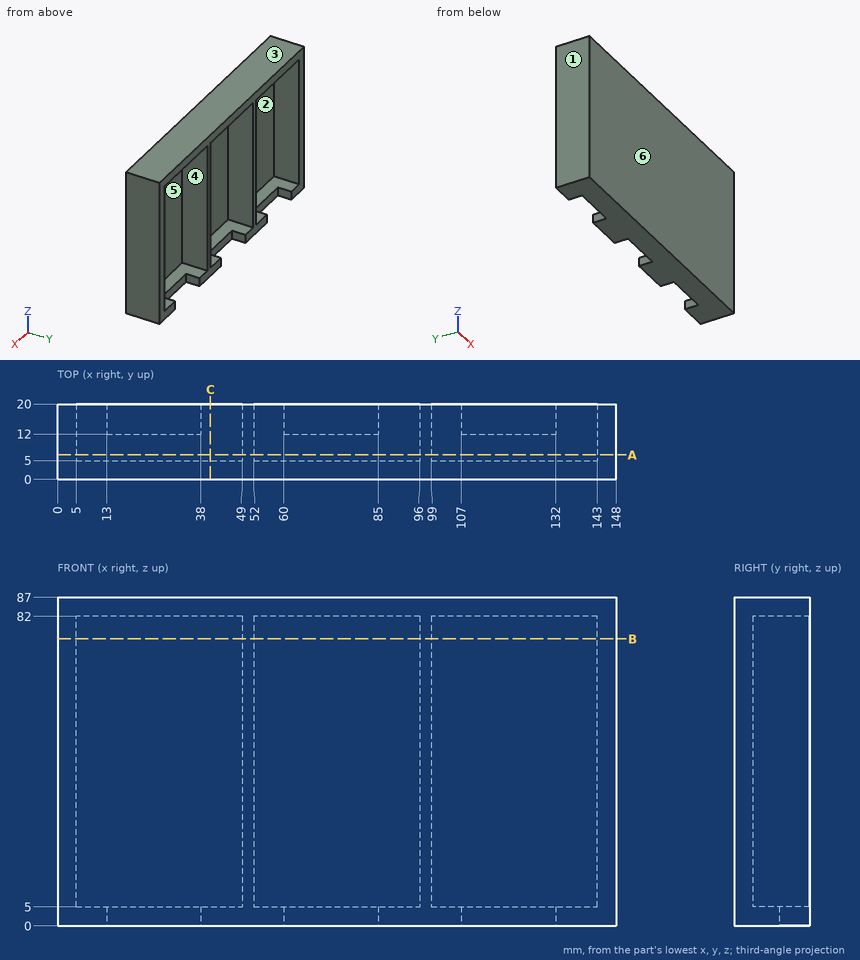
For this review, use the dimensioned drawing (mm, ordinates from the lowest corner) and the shaded views. A direction names the side the tool comes from. Round coordinates to 2 decimals unless told otherwise and drop trailing zeros. Write each loop counter-clockwise with the first axis right and the second up, starting at its lowest first coordinate (ties: lowest second). Pieces come first, ordered by that corner, then holes. Notation, with made-up numbers: (10, 79.25) -> (55, 79.25) arc R20 cw to (55, 111.25) -> close; hole circle Ø2 at (-1, -22). An arc over 180 degrees is marked (long way). Use one line per item in the form item = value.
Q1. The part is to be moulded in two halves that separate along Z. For the marked faces 1, 2, 3 and 4, say which applies: released by +Z, released by -Z, zero draft, split by the parting line, or undercut.
Resolved:
face_1 = zero draft
face_2 = undercut
face_3 = released by +Z
face_4 = undercut
Q2. Clearance check with flat-ended pins moving along their axes: pin 1 Ø5.5 at (y, z) = (15.5, 2) entering from -X; pin 2 Ø2 at (x, z) = (76, 74) entering from +Y; pin 3 Ø1.5 at (x, z) = (30, 2.5) entering from +Y. State where each tip first meets the part, or that it passes through.
Resolved:
pin_1 = 0
pin_2 = 5
pin_3 = 12
Q3. Consider section C-C (x = 40.5). State the section outline as (y, z) points.
Resolved:
outline = (0, 0) -> (20, 0) -> (20, 5) -> (5, 5) -> (5, 82) -> (20, 82) -> (20, 87) -> (0, 87) -> close
Q4. Consider section A-A (y = 6.5). State the section outline as (x, z) points, then the cut area to 3 significant figures.
Resolved:
outline = (0, 0) -> (148, 0) -> (148, 87) -> (0, 87) -> close; hole (5, 5) -> (49, 5) -> (49, 82) -> (5, 82) -> close; hole (52, 5) -> (96, 5) -> (96, 82) -> (52, 82) -> close; hole (99, 5) -> (143, 5) -> (143, 82) -> (99, 82) -> close
area = 2,710 mm²
Q5. To check wall thickness, follow probe 1 along X at (y, z) = (18, 21.5); probe 2 along Z at (x, y) = (19, 10); probe 3 along Y at (x, z) = (138, 75.5). State the ranges of each line that lie inside material, in increasing order. Write a range as from..to.
Resolved:
probe_1 = 0..5, 49..52, 96..99, 143..148
probe_2 = 0..5, 82..87
probe_3 = 0..5
Q6. Machinability: for the marked faces 5 and 6, which of the approach directions +Z, -Z, +X, -X, +Y, -Y give a long, thin tool a straight path to every point of the face, cutting with its end or side? Answer none if there is none.
Resolved:
face_5 = +Y
face_6 = +Z, -Z, +X, -X, -Y
Q7. Consider section B-B (z = 76). State the section outline as (x, y) points.
Resolved:
outline = (0, 0) -> (148, 0) -> (148, 20) -> (143, 20) -> (143, 5) -> (99, 5) -> (99, 20) -> (96, 20) -> (96, 5) -> (52, 5) -> (52, 20) -> (49, 20) -> (49, 5) -> (5, 5) -> (5, 20) -> (0, 20) -> close
